Job drawing, mm, ordinate dimensions from the low corner. One solid piece. Round coordinates to 2 decimals unless told otherwise and drop trailing zeros. Loops run counter-clockwise (first coordinate to the right, second up) from the corner with the lowest first, then second, coordinate; pieces in that order, holes last. Notation, with made-up numbers: M -21.5,16 L 27.5,16 A20 ccw 27.5,40 Z; hole C -26,0.5 d3. An arc over 180 degrees is marked long. Use one line per item in the form item = value.
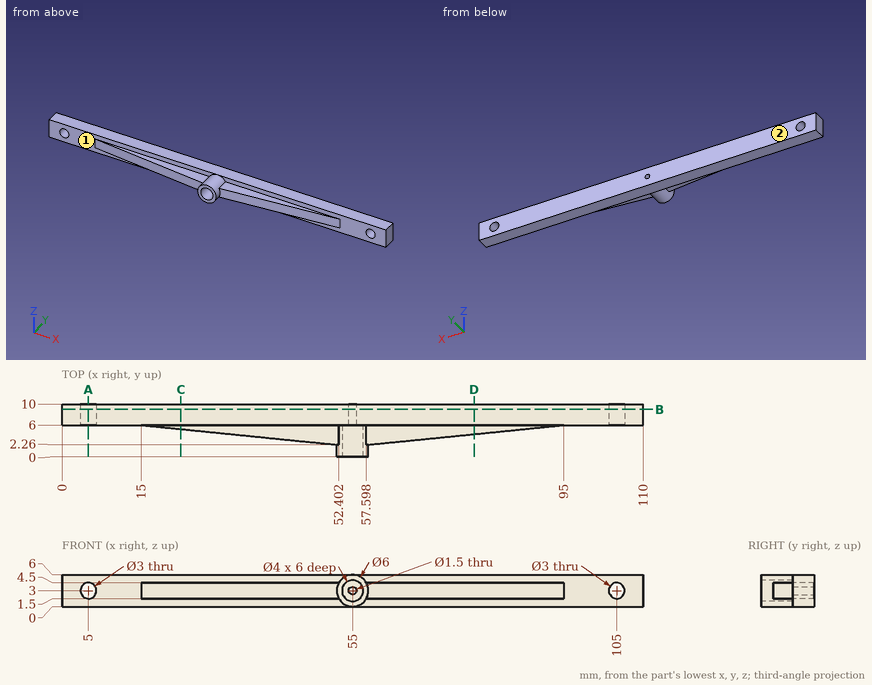
1. Cut at C-C on x = 22.5. Write the cut outline in (y, z).
Completed:
outline = M 5.25,1.5 L 6,1.5 L 6,0 L 10,0 L 10,6 L 6,6 L 6,4.5 L 5.25,4.5 Z
2. Cut at A-A on x = 5. Write the cut outline in (y, z).
Completed:
outline = M 6,0 L 10,0 L 10,1.5 L 6,1.5 Z; M 6,4.5 L 10,4.5 L 10,6 L 6,6 Z
3. Cut at B-B on y = 9. Write the cut outline in (x, z).
Completed:
outline = M 0,0 L 110,0 L 110,6 L 0,6 Z; hole C 5,3 d3; hole C 55,3 d1.5; hole C 105,3 d3
4. Drop flat-ended pins along their axis: P1, Ø3, axis at x = 55, z = 3, coming from the -Y side; P2, Ø3, axis at x = 55, z = 3, coming from the +Y side; P3, Ø3, axis at x = 26, y = 3.5, coming from the -Z side; P4, Ø1.5, axis at x = 64.5, z = 1, coming from the -Y side. Give the stop position or say it passes through.
Completed:
P1 = 6
P2 = 10
P3 = 1.5
P4 = 2.89
5. Cut at D-D on x = 78. Write the cut outline in (y, z), and give its area (3 significant figures).
Completed:
outline = M 4.3,1.5 L 6,1.5 L 6,0 L 10,0 L 10,6 L 6,6 L 6,4.5 L 4.3,4.5 Z
area = 29.1 mm2
6. Probe line 1 along Z through (x, y) = (105, 7.5); line 2 along Z through (x, y) = (55, 3.1); line 3 along X through (y, z) = (7.75, 2.5) (1 decimal). List the from-to ranges inside material, lowest first. Write a range as from..to.
Completed:
line_1 = 0..1.5, 4.5..6
line_2 = 0..1, 5..6
line_3 = 0..3.6, 6.4..54.4, 55.6..103.6, 106.4..110
7. Pull direction Y, two halves, no side cores. Call the marked faces 1 and 2: +Y half, -Y half, draft (parallel to the pull), parting line (faces both ways), or undercut.
Completed:
face_1 = -Y half
face_2 = +Y half
